from build123d import *

# Parameters (mm, degrees)
PAD005_DEPTH    = 30
SKETCH014_R     = 2
POCKET016_DEPTH = 5
FILLET001_R     = 2
FILLET002_R     = 15
FILLET003_R     = 7.9
FILLET004_R     = 10
FILLET005_R     = 2
SKETCH015_W     = 30.4
SKETCH015_H     = 30
POCKET017_DEPTH = 3.2
FILLET006_R     = 2
SKETCH020_R     = 0.8
POCKET021_DEPTH = 3


with BuildPart() as part:
    # Sketch013 → Pad005 (new body)
    with BuildSketch(Plane.XY):
        Polygon((-15, 30), (15, 30), (15, 25), (5, 25), (5, -25), (35, -25), (35, -30), (-35, -30), (-35, -25), (-5, -25), (-5, 25), (-15, 25), align=None)
    extrude(amount=PAD005_DEPTH)

    # Sketch014 (on Face11 of Pad005) → Pocket016 (cut)
    with BuildSketch(Plane(origin=(0, 25, 0), x_dir=(1, 0, 0), z_dir=(0, -1, 0))):
        with Locations((-10, 18.5)):
            Circle(SKETCH014_R)
        with Locations((10, 18.5)):
            Circle(SKETCH014_R)
        with Locations((10, 8.5)):
            Circle(SKETCH014_R)
        with Locations((-10, 8.5)):
            Circle(SKETCH014_R)
    extrude(amount=-POCKET016_DEPTH, mode=Mode.SUBTRACT)

    # Fillet001
    fillet001_edges = [part.edges().sort_by_distance(p)[0] for p in [
        (-5, 25, 15),
        (5, 25, 15),
    ]]
    fillet(fillet001_edges, radius=FILLET001_R)

    # Fillet002
    fillet002_edges = [part.edges().sort_by_distance(p)[0] for p in [
        (5, -25, 15),
        (-5, -25, 15),
    ]]
    fillet(fillet002_edges, radius=FILLET002_R)

    # Fillet003
    fillet003_edges = [part.edges().sort_by_distance(p)[0] for p in [
        (15, 27.5, 30),
        (15, 27.5, 0),
        (-15, 27.5, 30),
        (-15, 27.5, 0),
    ]]
    fillet(fillet003_edges, radius=FILLET003_R)

    # Fillet004
    fillet004_edges = [part.edges().sort_by_distance(p)[0] for p in [
        (-35, -27.5, 30),
        (-35, -27.5, 0),
        (35, -27.5, 30),
        (35, -27.5, 0),
    ]]
    fillet(fillet004_edges, radius=FILLET004_R)

    # Fillet005
    fillet005_edges = [part.edges().sort_by_distance(p)[0] for p in [
        (5, 6.5, 30),
        (-5, 6.5, 30),
    ]]
    fillet(fillet005_edges, radius=FILLET005_R)

    # Sketch015 (on Face4 of Fillet005) → Pocket017 (cut)
    with BuildSketch(Plane(origin=(0, -30, 0), x_dir=(1, 0, 0), z_dir=(0, -1, 0))):
        with Locations((0, 15)):
            Rectangle(SKETCH015_W, SKETCH015_H)
    extrude(amount=-POCKET017_DEPTH, mode=Mode.SUBTRACT)

    # Fillet006
    fillet006_edges = [part.edges().sort_by_distance(p)[0] for p in [
        (15.2, -26.8, 15),
        (-15.2, -26.8, 15),
    ]]
    fillet(fillet006_edges, radius=FILLET006_R)

    # Sketch020 (on Face5 of Fillet006) → Pocket021 (cut)
    with BuildSketch(Plane(origin=(0, -26.8, 0), x_dir=(1, 0, 0), z_dir=(0, -1, 0))):
        with Locations((0, 15)):
            Circle(SKETCH020_R)
    extrude(amount=-POCKET021_DEPTH, mode=Mode.SUBTRACT)


with BuildPart() as part_1:
    # Body002 placement: moved
    add(part.part.moved(Location((-0.28, -65.8, -23.42))))


solid = part_1.part
The listing builds one solid part. Answer for the finished solid, in the listing's coordinates (mm). A direction names the side the tool comes from. Coordinates: 2 decimals unless noted, no trailing zeros. Loops run counter-clockwise (first coordinate to the right, second up) from the corner with the lowest first, then second, coordinate; pieces in that order, holes last. Notation, with made-up numbers: M 84,21 L 113,21 A24 cw 113,60 Z; hole C -1.5,31 d8. An arc over 180 degrees is marked long. Answer in a Markdown table with one row per item.
1) Find section C-C (y = -46.5). Determine the outline of the cut face in (x, z).
Answers below:
| item | result |
|---|---|
| outline | M -5.28,-21.42 A2 ccw -3.28,-23.42 L 2.72,-23.42 A2 ccw 4.72,-21.42 L 4.72,4.58 A2 ccw 2.72,6.58 L -3.28,6.58 A2 ccw -5.28,4.58 Z |
2) Given pin 1 (5 mm diameter, centred on x = 9.72, z = -4.92, fed in from -Y); pin 2 (13 mm diameter, centred on y = -57, z = -4, fed in from +X); pin 3 (3.5 mm diameter, centred on y = -37.5, z = -8, fed in from -X), each flat-ended and moving along its own axis, determine where each tip first touches the part or whether it passes through.
Answers below:
| item | result |
|---|---|
| pin 1 | y = -92.6 |
| pin 2 | x = 4.72 |
| pin 3 | x = -15.28 |
3) Determine the mould class of faces 5 (the cylindrical face through (22.18, -91.37, -22.82)), 6 (the cylindrical face through (4.15, -59.53, 5.98)), 7 (the flat face through (-35.28, -94, -8)) for opening direction Y: released by +Y, released by -Y, zero draft, split by the parting line, or undercut.
Answers below:
| item | result |
|---|---|
| face 5 | released by +Y |
| face 6 | undercut |
| face 7 | zero draft |
4) Find section A-A (z = -4.92). Count the separate pieces of the cut face and the enclosed holes in it, then the cut area to 3 significant figures.
Answers below:
| item | result |
|---|---|
| separate pieces | 3 |
| enclosed holes | 0 |
| area | 959 mm^2 |
5) Find the intervals of material crossed by probe 1 along X at (y, z) = (-39, -15); probe 2 along X at (y, z) = (-39, -14); probe 3 along Z at (x, y) = (-0.28, -90.45), in increasing order.
Answers below:
| item | result |
|---|---|
| probe 1 | -15.27 to -12.28, -8.28 to 7.72, 11.72 to 14.71 |
| probe 2 | -15.27 to -12.06, -8.5 to 7.94, 11.5 to 14.71 |
| probe 3 | -23.42 to -9.22, -7.62 to 6.58 |
6) Which of the six approach directions +Z, -Z, +X, -X, +Y, -Y give full straight-line access (tool end or side, diameter ignored) to faces 1 (the cylindrical face through (12.34, -37.32, -21.17)), 2 (the flat face through (4.72, -59, -9)), 3 (the flat face through (-3, -92.6, -8)), 4 (the cylindrical face through (-14.68, -40.23, -8.52))?
Answers below:
| item | result |
|---|---|
| face 1 | -Z, +X, +Y |
| face 2 | +Z, -Z, +X |
| face 3 | +Z, -Z, -Y |
| face 4 | +Z, -Z, -X |
7) Find section D-D (x = -22.5). Determine the outline of the cut face in (y, z).
Answers below:
| item | result |
|---|---|
| outline | M -95.8,-23.42 L -92.8,-23.42 A2 ccw -90.8,-21.42 L -90.8,4.58 A2 ccw -92.8,6.58 L -95.8,6.58 Z |
